Design review of the part built by this model. Coordinates are the model's own, in mm. A direction names the side the tool comes from. Give positions to 0.01 mm unless a question says otherwise; leave off trailing zeros. Loops run counter-clockwise (first coordinate to the right, second up) from the corner with the lowest first, then second, coordinate; pieces in that order, holes last. Notation, with made-up numbers: (54.25, 46.25) - (95.25, 46.25) arc R20 ccw to (95.25, 58.25) - close; hole circle Ø4 at (20.5, 8.25). An arc over 180 degrees is marked (long way). One line per item, written item: value. Start each with the question number.
Autodesk Fusion 360 part; units mm, degrees
sketch "Skizze1" plane through (0, 0, 0) normal (0, 0, 1) x (1, 0, 0)
  line L0 (0, 0) -> (-57, 0)
  line L1 (-57, 0) -> (-57, 28)
  line L2 (-57, 28) -> (0, 28)
  line L3 (0, 28) -> (0, 0)
  line L4 (-57, 23) -> (-63, 23)
  line L5 (-63, 23) -> (-63, 5)
  line L6 (-63, 5) -> (-57, 5)
  line L7 (-57, 5) -> (-57, 23)
  line L8 (0, 14) -> (-57, 14) construction
  dimension "d1" = 57
  dimension "d2" = 28
  dimension "d3" = 6
  dimension "d4" = 18
extrude "Extrusion1" add sketch "Skizze1" along normal blind 1.6
sketch "Skizze2" plane through (0, 0, 0) normal (1, 0, 0) x (0, 1, 0)
  line L0 (0, 0) -> (28, 0)
  line L1 (28, 0) -> (28, 1.6)
  line L2 (28, 1.6) -> (0, 1.6)
  line L3 (0, 1.6) -> (0, 0)
  line L4 (23, 1.6) -> (5, 1.6)
  line L5 (5, 1.6) -> (0, 1.6)
  line L6 (0, 1.6) -> (28, 1.6)
  line L7 (28, 1.6) -> (23, 1.6)
  line L8 (5.1, 4.8) -> (10.9, 4.8)
  line L9 (10.9, 1.6) -> (5.1, 1.6)
  line L10 (17.1, 4.8) -> (22.9, 4.8)
  line L11 (17.1, 1.6) -> (22.9, 1.6)
  arc A0 (5.1, 4.8) -> (5.1, 1.6) centre (5.1, 3.2) ccw
  arc A1 (10.9, 1.6) -> (10.9, 4.8) centre (10.9, 3.2) ccw
  arc A2 (17.1, 4.8) -> (17.1, 1.6) centre (17.1, 3.2) ccw
  arc A3 (22.9, 1.6) -> (22.9, 4.8) centre (22.9, 3.2) ccw
  line L12 (14, 1.6) -> (14, 0) construction
  dimension "d7" = 3.2
  dimension "d8" = 3.2
  dimension "d9" = 5.8
  dimension "d10" = 5.8
  dimension "d11" = 6.2
extrude "Extrusion2" add sketch "Skizze2" against normal blind 7.3 contours L2 L4 L6 L8 L9 A0 A1 | L2 L4 L6 L10 L11 A2 A3
sketch "Skizze3" plane through (0, 0, 0) normal (0, 0, -1) x (1, 0, 0)
  line L0 (-63, -23) -> (-57, -23)
  line L1 (-57, -23) -> (-57, -28)
  line L2 (-57, -28) -> (0, -28)
  line L3 (0, -28) -> (0, 0)
  line L4 (0, 0) -> (-57, 0)
  line L5 (-57, 0) -> (-57, -5)
  line L6 (-57, -5) -> (-63, -5)
  line L7 (-63, -5) -> (-63, -23)
  line L8 (0, -26.7) -> (-57, -26.7) construction
  line L9 (0, -1.3) -> (-57, -1.3) construction
  line L10 (-1.83, -26.7) -> (-1.83, -1.3) construction
  line L11 (-55.17, -26.7) -> (-55.17, -1.3) construction
  line L12 (-1.83, -26.7) -> (0, -26.7) construction
  line L13 (-57, -26.7) -> (-55.17, -26.7) construction
  line L14 (0, -14) -> (-63, -14) construction
  point P0 (-1.83, -1.3)
  point P1 (-55.17, -1.3)
  point P2 (-55.17, -26.7)
  point P3 (-1.83, -26.7)
  dimension "d14" = 53.34
  dimension "d16" = 25.4
equation "d8 = d7"
equation "d9 = d10"
equation "d10 = 9 mm - 3.2 mm"
equation "d11 = 3 mm + 3.2 mm"
equation "d14 = ( 21 * 2.54 ) * 1 mm"
equation "d16 = ( 10 * 2.54 ) * 1 mm"
(1) Take a section at D-D on y = 25.5. State the section outline as (x, z) points.
(2) For pin 1 Ø0.8 at (x, z) = (-61, 0.5) entering from -Y; pin 2 Ø2.5 at (y, z) = (22, 4) entering from -X; pin 3 Ø1.8 at (y, z) = (1.5, 1) entering from -X, all flat-tipped, find the tip position at first contact; note any pin that passes through.
(3) Take a section at B-B on y = 20.5. State the section outline as (x, z) points, and give its area (3 significant figures).
(4) Take a section at C-C on x = -27.5. State the section outline as (y, z) points.
(5) Take a section at A-A on z = 3.15. State the section outline as (x, y) points, and give its area (3 significant figures).
(6) To check wall thickness, follow L1, parallel to Z at x = -30.5, y = 15.25; L2, parallel to X at y = 24, z = 4.2; L3, parallel to X at y = 24.75, z = 0.95. State the ranges of each line that lie inside material, in increasing order. Write a range as from..to.
(7) Machinability: for faces 4 (the flat face through (-57, 25, 1)), 5 (the flat face through (-7.3, 8, 3)), 6 (the flat face through (-60, 5, 1)), 7 (the flat face through (-29, 28, 1)), which of the approach directions +Z, -Z, +X, -X, +Y, -Y give a long, thin tool a straight path to every point of the face, cutting with its end or side? Answer none if there is none.
(8) Draft analysis for pull direction Y (two halves, no side actions). For faces 1 (the cylindrical face through (-3.6, 15.5, 3.2)), 2 (the flat face through (-60, 23, 1)), 3 (the flat face through (-57, 2, 1)), state which applies: pulls with the +Y half, pulls with the -Y half, needs draft (parallel to the pull), parting line crosses it, or undercut.
Here are the results:
1. outline: (-57, 0) - (0, 0) - (0, 1.6) - (-57, 1.6) - close
2. pin 1: y = 5
2. pin 2: x = -7.3
2. pin 3: x = -57
3. outline: (-63, 0) - (0, 0) - (0, 4.8) - (-7.3, 4.8) - (-7.3, 1.6) - (-63, 1.6) - close
3. area: 124 mm²
4. outline: (0, 0) - (28, 0) - (28, 1.6) - (0, 1.6) - close
5. outline: (-7.3, 3.5) - (0, 3.5) - (0, 12.5) - (-7.3, 12.5) - close; (-7.3, 15.5) - (0, 15.5) - (0, 24.5) - (-7.3, 24.5) - close
5. area: 131 mm²
6. L1: 0..1.6
6. L2: -7.3..0
6. L3: -57..0
7. face 4: +Z, -Z, -X, +Y
7. face 5: +Z, -X, +Y, -Y
7. face 6: +Z, -Z, -X, -Y
7. face 7: +Z, -Z, +X, -X, +Y
8. face 1: undercut
8. face 2: pulls with the +Y half
8. face 3: needs draft
